For this review, take the finished solid that the model builds, in its own axes (mm). A direction names the side the tool comes from. Coordinates: 2 decimals unless noted, no trailing zeros. Loops run counter-clockwise (first coordinate to the right, second up) from the corner with the lowest first, then second, coordinate; pieces in that order, holes last.
1. Take a section at B-B, the plane y = 0. State the section outline as (x, z) points (3 decimals), then the cut area to 3 significant figures.
2. Take a section at A-A, the plane x = 0. State the section outline as (y, z) points (3 decimals), then the cut area to 3 significant figures.
3. Take a section at C-C, the plane z = 23.5. State the section outline as (x, y) points (3 decimals), then the cut area to 3 significant figures.
4. To check wall thickness, follow probe 1 along Y at (x, z) = (49, 33) (3 decimals); probe 2 along Z at (x, y) = (55.5, -12); probe 3 along Z at (x, y) = (-2, -21). State the ranges of each line that lie inside material, in increasing order.
5. Clearance check with flat-ended pins moving along their axes: P1, Ø8, axis at x = 52, z = 15, coming from the -Y side (3 decimals); P2, Ø8.5, axis at x = 14.14, y = 14.14, coming from the +Z side; P3, Ø5, axis at x = -14.14, y = -14.14, coming from the -Z side; P4, Ø2, axis at x = 33.5, z = 8.5, coming from the -Y side. State where each tip first meets the part, or that it passes through.
6. Take a section at D-D, the plane x = 27. State the section outline as (y, z) points.
7. Mouldability with a two-part tool opening along X and no side actions: class faces 1 (the face through (46.575, 0, 38)), 2 (the face through (57, 0, 47.5)), 3 (the face through (0, -16.155, -1)) as pulls with the +X half, pulls with the -X half, needs draft (parallel to the pull), parting line crosses it, or undercut.
8. Machinability: for faces 4 (the face through (-3, -15, -1)), 5 (the face through (58.54, 13.6, 34.35)), 6 (the face through (58.54, -13.6, 40.5)), 7 (the face through (46.575, 0, 11)), 8 (the face through (31.55, -9.93, 20.53)), which of the approach directions +Z, -Z, +X, -X, +Y, -Y give a long, thin tool a straight path to every point of the face, cutting with its end or side? Answer none if there is none.
Autodesk Inventor part; units mm, degrees
ref_plane "工作平面6" through (38.7456, -15.075, 50.5) normal (0, -1, 0) x (1, 0, 0)
ref_plane "工作平面7" through (38.7456, -15.075, 50.5) normal (0, -1, 0) x (1, 0, 0)
ref_plane "YZ Plane" through (0, 0, 0) normal (1, 0, 0) x (0, 1, 0)
sketch "草圖1" plane through (0, 0, 0) normal (0, 0, 1) x (1, 0, 0)
  circle A0 centre (0, 0) radius 19.6
  circle A1 centre (0, 0) radius 41.575
  dimension "d0" = 39.2
  dimension "d1" = 83.15
extrude "擠出1" add sketch "草圖1" along normal blind 5
sketch "草圖2" plane through (0, 0, 0) normal (0, 0, -1) x (-1, 0, 0)
  circle A0 centre (0, 0) radius 41.575
extrude "擠出2" add sketch "草圖2" along normal blind 4
sketch "草圖4" plane through (0, 0, 5) normal (0, 0, 1) x (1, 0, 0)
  circle A0 centre (0, 0) radius 41.575
  circle A1 centre (0, 0) radius 37.575
  dimension "d14" = 4
extrude "擠出4" add sketch "草圖4" along normal blind 47.5
sketch "草圖5" plane through (0, 0, 5) normal (0, 0, 1) x (1, 0, 0)
  circle A0 centre (0, 0) radius 37.575
  circle A1 centre (0, 0) radius 33.075
  dimension "d17" = 4.5
extrude "擠出5" add sketch "草圖5" along normal blind 31.5
sketch "草圖6" plane through (0, 0, -4) normal (0, 0, -1) x (-1, 0, 0)
  line L0 (-66.575, 15.075) -> (-66.575, -15.075)
  line L1 (-66.575, 15.075) -> (-38.7456, 15.075)
  circle A0 centre (0, 0) radius 41.575
  line L2 (-66.575, -15.075) -> (-38.7456, -15.075)
  point P0 (-41.575, 0)
  dimension "d20" = 30.15
  dimension "d22" = 15.075
  dimension "d25" = 25
extrude "擠出6" add sketch "草圖6" against normal up to surface (56.5 mm away) contours L1 A0 L2 L0
sketch "草圖7" plane through (66.575, -15.075, -4) normal (1, 0, 0) x (0, 0, -1)
  line L0 (-56.5, 30.15) -> (-56.5, 0)
  line L1 (0, 0) -> (-56.5, 0)
  line L2 (0, 30.15) -> (0, 0)
  line L3 (0, 30.15) -> (-56.5, 30.15)
  line L4 (-51.5, 5) -> (-31.35, 5)
  line L5 (-31.35, 5) -> (-31.35, 25.15)
  line L6 (-31.35, 25.15) -> (-51.5, 25.15)
  line L7 (-51.5, 25.15) -> (-51.5, 5)
  line L8 (-51.5, 5) -> (-31.35, 25.15) construction
  line L9 (-31.35, 5) -> (-51.5, 25.15) construction
  line L10 (-25.15, 5.0185) -> (-5, 5.0185)
  line L11 (-5, 5.0185) -> (-5, 25.15)
  line L12 (-5, 25.15) -> (-25.15, 25.15)
  line L13 (-25.15, 25.15) -> (-25.15, 5.0185)
  line L14 (-25.15, 5.0185) -> (-5, 25.15) construction
  line L15 (-5, 5.0185) -> (-25.15, 25.15) construction
  point P0 (-4, 15.075)
  point P1 (-41.425, 15.075)
  point P2 (-15.075, 15.0842)
  dimension "d26" = 20.15
  dimension "d27" = 20.15
  dimension "d28" = 20.15
  dimension "d29" = 5
  dimension "d30" = 5
  dimension "d31" = 5
extrude "擠出7" cut sketch "草圖7" against normal blind 20 contours L7 L6 L5 L4 | L13 L12 L11 L10
sketch "草圖8" plane through (0, 0, 52.5) normal (0, 0, 1) x (1, 0, 0)
  line L0 (52.9465, -6.0747) -> (44.9865, -6.0635)
  line L1 (52.9465, -6.0747) -> (52.9551, 0.0253)
  line L2 (44.9951, 0.0365) -> (52.9551, 0.0253)
  line L3 (44.9865, -6.0635) -> (44.9951, 0.0365)
  circle A0 centre (48.975, -7.075) radius 2.165
  circle A1 centre (48.975, 7.075) radius 2.165
  line L4 (38.7456, -15.075) -> (66.575, -15.075)
  line L5 (66.575, 15.075) -> (40.0902, 15.075)
  point P0 (0, 0)
  dimension "d36" = 4.33
  dimension "d37" = 4.33
  dimension "d38" = 8
  dimension "d39" = 8
extrude "擠出8" cut sketch "草圖8" against normal up to surface (5 mm away) contours A0 L0 | L0 A0 | A1
ref_plane "工作平面6" through (38.7456, -15.075, 50.5) normal (0, -1, 0) x (1, 0, 0)
sketch "草圖9" plane through (38.7456, -15.075, 50.5) normal (0, -1, 0) x (1, 0, 0)
  line L0 (27.8294, -29.35) -> (27.8294, -49.5)
  line L1 (27.8294, -29.35) -> (7.8294, -29.35)
  line L2 (7.8294, -29.35) -> (7.8294, -49.5)
  line L3 (27.8294, -49.5) -> (7.8294, -49.5)
  line L4 (27.8294, -3) -> (27.8294, -23.15)
  line L5 (27.8294, -3) -> (7.8294, -3)
  line L6 (7.8294, -3) -> (7.8294, -23.15)
  line L7 (27.8294, -23.15) -> (7.8294, -23.15)
  circle A0 centre (17.8294, -39.425) radius 2.1
  circle A1 centre (17.8294, -13.075) radius 2.1
  point P0 (-38.7456, -50.5)
  dimension "d42" = 4.2
  dimension "d43" = 4.2
extrude "擠出9" cut sketch "草圖9" against normal through all contours A0 | A1
ref_plane "工作平面7" through (38.7456, -15.075, 50.5) normal (0, -1, 0) x (1, 0, 0)
sketch "草圖10" plane through (38.7456, -15.075, 50.5) normal (0, -1, 0) x (1, 0, 0)
  circle A0 centre (17.8294, -39.425) radius 2.1
  circle A1 centre (17.8294, -39.425) radius 3.65
  circle A2 centre (17.8294, -13.075) radius 2.1
  circle A3 centre (17.8294, -13.075) radius 3.65
  point P0 (-38.7456, -50.5)
  dimension "d46" = 7.3
  dimension "d47" = 7.3
extrude "擠出10" cut sketch "草圖10" against normal blind 3
sketch "草圖14" plane through (0, 0, 5) normal (0, 0, 1) x (1, 0, 0)
  circle A0 centre (0, 0) radius 19.6
extrude "擠出13" add sketch "草圖14" against normal up to surface (9 mm away)
sketch "草圖19" plane through (0, 0, -4) normal (0, 0, -1) x (-1, 0, 0)
  arc A0 (-38.7456, -15.075) -> (-38.7456, 15.075) centre (0, 0) ccw
  line L0 (-38.7456, 15.075) -> (-66.575, 15.075)
  line L1 (-66.575, 15.075) -> (-66.575, -15.075)
  line L2 (-66.575, -15.075) -> (-38.7456, -15.075)
extrude "擠出18" add sketch "草圖19" along normal blind 2
sketch "草圖20" plane through (0, 0, -6) normal (0, 0, -1) x (-1, 0, 0)
  circle A0 centre (0, 0) radius 20 construction
  line L0 (0, 0) -> (14.1421, -14.1421) construction
  line L1 (0, 0) -> (20, 0) construction
  circle A1 centre (14.1421, -14.1421) radius 3.275
  circle A2 centre (14.1421, 14.1421) radius 3.275
  circle A3 centre (-14.1421, 14.1421) radius 3.275
  circle A4 centre (-14.1421, -14.1421) radius 3.275
  circle A5 centre (0, 0) radius 33.075
  circle A6 centre (0, 0) radius 14.075
  line L2 (3, -16.1547) -> (-3, -16.1547)
  line L3 (-3, -16.1547) -> (-3, -13.7516)
  line L4 (3, -16.1547) -> (3, -13.7516)
  line L5 (16.1547, 3) -> (13.7516, 3)
  line L6 (16.1547, -3) -> (13.7516, -3)
  line L7 (16.1547, 3) -> (16.1547, -3)
  line L8 (-3, 16.1547) -> (-3, 13.7516)
  line L9 (3, 16.1547) -> (3, 13.7516)
  line L10 (-3, 16.1547) -> (3, 16.1547)
  line L11 (-16.1547, -3) -> (-13.7516, -3)
  line L12 (-16.1547, 3) -> (-13.7516, 3)
  line L13 (-16.1547, -3) -> (-16.1547, 3)
  dimension "d83" = 40
  dimension "d84" = 45
  dimension "d85" = 6.55
  dimension "d88" = 360
  dimension "d90" = 28.15
  dimension "d91" = 6
  dimension "d92" = 3
  dimension "d95" = 360
extrude "擠出19" cut sketch "草圖20" against normal up to surface (11 mm away) contours A1 | A2 | A3 | A4 | A6 | A6 L5 L7 L6 | A6 L8 L10 L9 | L4 L2 L3 A6 | A6 L11 L13 L12
mirror "鏡射2" about plane through (0, 0, 0) normal (0, 1, 0) of "擠出10"
equation "\"d27\" = d26"
equation "\"d28\" = d26"
properties part number "j2 moving part option2_3D 列印"
Results list:
1. outline: (-41.575, -6) - (-16.155, -6) - (-16.155, 5) - (-33.075, 5) - (-33.075, 36.5) - (-37.575, 36.5) - (-37.575, 52.5) - (-41.575, 52.5) - close; (16.155, -6) - (66.575, -6) - (66.575, 1) - (46.575, 1) - (46.575, 21.15) - (66.575, 21.15) - (66.575, 27.35) - (46.575, 27.35) - (46.575, 47.5) - (66.575, 47.5) - (66.575, 52.5) - (37.575, 52.5) - (37.575, 36.5) - (33.075, 36.5) - (33.075, 5) - (16.155, 5) - close
1. area: 1,880 mm2
2. outline: (-41.575, -6) - (-16.155, -6) - (-16.155, 5) - (-33.075, 5) - (-33.075, 36.5) - (-37.575, 36.5) - (-37.575, 52.5) - (-41.575, 52.5) - close; (16.155, -6) - (41.575, -6) - (41.575, 52.5) - (37.575, 52.5) - (37.575, 36.5) - (33.075, 36.5) - (33.075, 5) - (16.155, 5) - close
2. area: 1,220 mm2
3. outline: (38.746, -15.075) - (66.575, -15.075) - (66.575, 15.075) - (38.746, 15.075) arc R41.575 ccw (long way) to start; hole circle Ø66.15 at (0, 0)
3. area: 2,780 mm2
4. probe 1: y = -15.075 to -10.075, 10.075 to 15.075
4. probe 2: z = -6 to 9.27, 12.88 to 35.62, 39.23 to 52.5
4. probe 3: z = -6 to 5
5. P1: stops at y = -15.075
5. P2: stops at z = 5
5. P3: passes through
5. P4: stops at y = -25.93
6. outline: (-31.61, -6) - (31.61, -6) - (31.61, 52.5) - (26.13, 52.5) - (26.13, 36.5) - (19.1, 36.5) - (19.1, 5) - (-19.1, 5) - (-19.1, 36.5) - (-26.13, 36.5) - (-26.13, 52.5) - (-31.61, 52.5) - close
7. face 1: pulls with the +X half
7. face 2: needs draft
7. face 3: undercut
8. face 4: +Z, -Z
8. face 5: +Y
8. face 6: -Y
8. face 7: +X
8. face 8: +Z
